Here's how the part is built. I have some questions about the finished solid (model axes, mm). Face numbers are marked on the shaded views. Give positions to 0.01 mm unless a question says otherwise; leave off trailing zeros. Write each loop counter-clockwise with the first axis right and the second up, starting at its lowest first coordinate (ties: lowest second). Pieces come first, ordered by that corner, then holes. Notation, with made-up numbers: (-12.5, 25.25) -> (-4.5, 25.25) arc R18 cw to (-4.5, 31.25) -> close; hole circle Ø10 at (60.5, 47). An arc over 180 degrees is marked (long way). Use CSV: the item, a comma, the result in double quotes. Start each with the question number.
(1) Suppose I cut it at D-D on z = -30. List the corners of the cut face in (x, y) for me (3 decimals), plus the area to 3 significant figures.
(2) Suppose I cut it at B-B on z = -66.56. List the corners of the cut face in (x, y) for me (3 decimals).
(3) If we mould it in two halves opening along Z, with no side actions, what happens to the marked faces 1 and 2? For each: pulls with the +Z half, pulls with the -Z half, needs draft (parallel to the pull), parting line crosses it, or undercut.
(4) For pin 1 Ø13 at (y, z) = (191.5, -9.5) entering from +X; pin 2 Ø4.5 at (x, y) = (22.5, 211.5) entering from -Z (3 decimals); pin 3 Ø6 at (x, z) = (10.165, -66.56) entering from +Y, each with a flat end and sliding along its axis, tell me the tip position at first contact or that it passes through.
(5) Suppose I cut it at A-A on y = 120. List the corners of the cut face in (x, z) for me (1 decimal), plus the area to 3 significant figures.
(6) I need wall thicknesses on L1, parallel to Z at x = 25, y = 84.5 (3 decimals); L2, parallel to Z at x = 8.75, y = 285; L3, parallel to X at y = 20.5, z = -35.5 (3 decimals). Which ranges of each line are inside material? Lowest first, please. Write a range as [from, to].
(7) Suppose I cut it at C-C on y = 25.5. List the corners of the cut face in (x, z) for me (3 decimals), plus the area to 3 significant figures.
from build123d import *

# Parameters (mm, degrees)
BOSS_EXTRUDE1_DEPTH = 300
SKETCH3_R           = 5
CUT_EXTRUDE1_DEPTH  = 329.551266015
SKETCH5_R           = 5
CUT_EXTRUDE2_DEPTH  = 10
SKETCH7_R           = 5
CUT_EXTRUDE5_DEPTH  = 10


with BuildPart() as part:
    # Sketch2 → Boss-Extrude1 (new body)
    with BuildSketch(Plane(origin=(0, 0, 0), x_dir=(1, 0, 0), z_dir=(0, 1, 0))):
        Polygon((0, 0), (0, 133.12), (15, 133.12), (15, 116.725), (27, 116.725), (27, 111.06), (17.665, 111.06), (17.665, 22.06), (27, 22.06), (27, 16.395), (15, 16.395), (15, 0), align=None)
    extrude(amount=BOSS_EXTRUDE1_DEPTH)

    # Sketch3 → Cut-Extrude1 (cut, through all)
    with BuildSketch(Plane(origin=(15, 0, 0), x_dir=(0, 0, -1), z_dir=(1, 0, 0))):
        with Locations((8.1975, 285)):
            Circle(SKETCH3_R)
        with Locations((8.1975, 230)):
            Circle(SKETCH3_R)
        with Locations((8.1975, 175)):
            Circle(SKETCH3_R)
        with Locations((8.1975, 120)):
            Circle(SKETCH3_R)
        with Locations((8.1975, 65)):
            Circle(SKETCH3_R)
        with Locations((8.1975, 10)):
            Circle(SKETCH3_R)
        with Locations(Location((124.9225, 10, 0), (0, 0, 180))):
            Circle(SKETCH3_R)
        with Locations(Location((124.9225, 65, 0), (0, 0, 180))):
            Circle(SKETCH3_R)
        with Locations(Location((124.9225, 120, 0), (0, 0, 180))):
            Circle(SKETCH3_R)
        with Locations(Location((124.9225, 175, 0), (0, 0, 180))):
            Circle(SKETCH3_R)
        with Locations(Location((124.9225, 230, 0), (0, 0, 180))):
            Circle(SKETCH3_R)
        with Locations(Location((124.9225, 285, 0), (0, 0, 180))):
            Circle(SKETCH3_R)
    extrude(amount=-CUT_EXTRUDE1_DEPTH, mode=Mode.SUBTRACT)

    # Sketch5 → Cut-Extrude2 (cut)
    with BuildSketch(Plane(origin=(0, 300, 0), x_dir=(1, 0, 0), z_dir=(0, 1, 0))):
        with Locations(Location((10.165, 66.563164806, 0), (0, 0, 270))):
            Circle(SKETCH5_R)
    extrude(amount=-CUT_EXTRUDE2_DEPTH, mode=Mode.SUBTRACT)

    # Sketch7 → Cut-Extrude5 (cut)
    with BuildSketch(Plane.XZ):
        with Locations(Location((10.165, -66.56, 0), (0, 0, 270))):
            Circle(SKETCH7_R)
    extrude(amount=-CUT_EXTRUDE5_DEPTH, mode=Mode.SUBTRACT)


solid = part.part
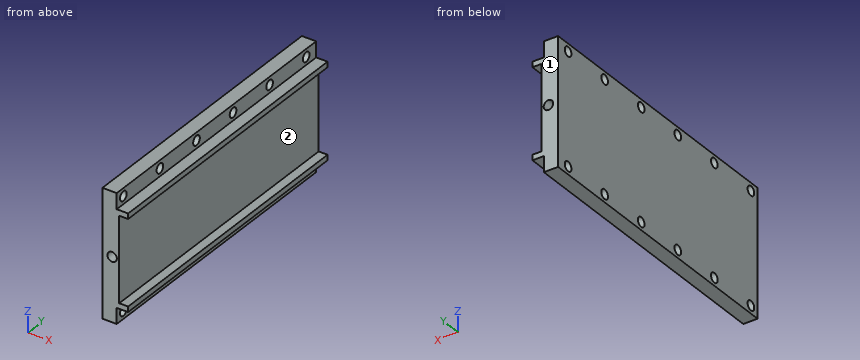
Geometry says:
1,outline,"(0, 0) -> (17.665, 0) -> (17.665, 300) -> (0, 300) -> close"
1,area,"5,300 mm²"
2,outline,"(0, 0) -> (5.165, 0) -> (5.165, 10) -> (15.165, 10) -> (15.165, 0) -> (17.665, 0) -> (17.665, 300) -> (15.165, 300) -> (15.165, 290) -> (5.165, 290) -> (5.165, 300) -> (0, 300) -> close"
3,face 1,"needs draft"
3,face 2,"undercut"
4,pin 1,"x = 15"
4,pin 2,"z = -116.725"
4,pin 3,"y = 290"
5,outline,"(0, -133.1) -> (15, -133.1) -> (15, -129.9) -> (0, -129.9) -> close; (0, -119.9) -> (15, -119.9) -> (15, -116.7) -> (27, -116.7) -> (27, -111.1) -> (17.7, -111.1) -> (17.7, -22.1) -> (27, -22.1) -> (27, -16.4) -> (15, -16.4) -> (15, -13.2) -> (0, -13.2) -> close; (0, -3.2) -> (15, -3.2) -> (15, 0) -> (0, 0) -> close"
5,area,"2,070 mm²"
6,L1,"[-116.725, -111.06], [-22.06, -16.395]"
6,L2,"[-133.12, -129.92], [-119.92, -13.2], [-3.2, 0]"
6,L3,"[0, 17.665]"
7,outline,"(0, -133.12) -> (15, -133.12) -> (15, -116.725) -> (27, -116.725) -> (27, -111.06) -> (17.665, -111.06) -> (17.665, -22.06) -> (27, -22.06) -> (27, -16.395) -> (15, -16.395) -> (15, 0) -> (0, 0) -> close"
7,area,"2,370 mm²"
